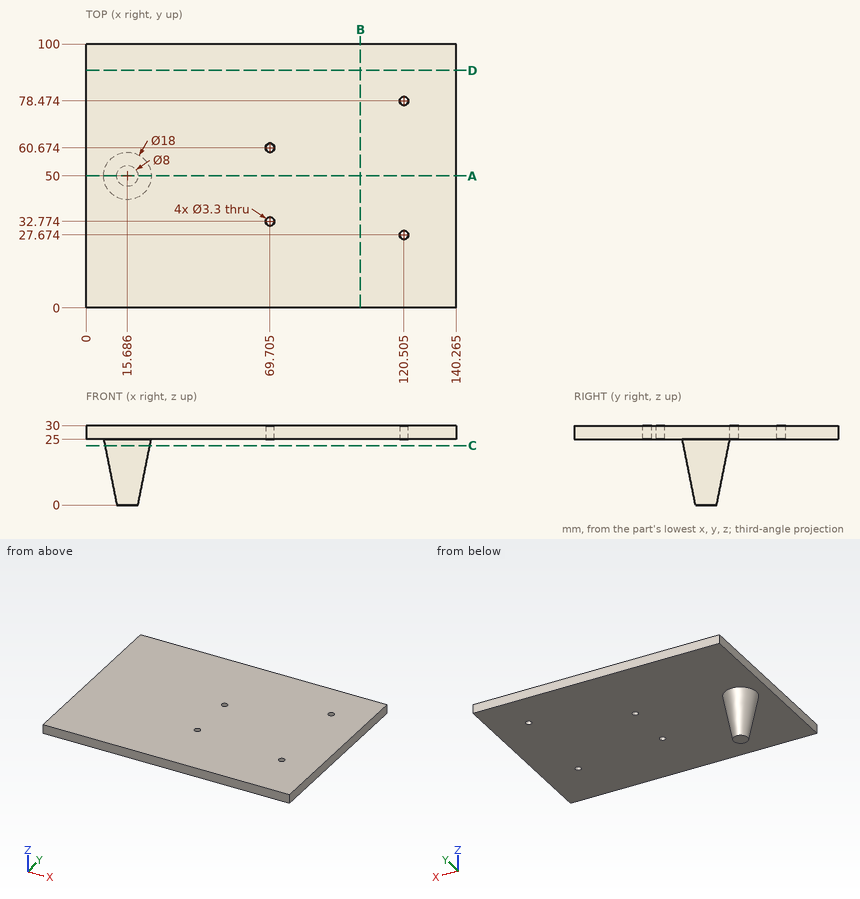
Geometry: see drawing. Coordinates: mm, zero at the bounding-box minimum. Give positions to 0.01 mm unless a question says otherwise; leave off trailing zeros. Order: outer loops, then holes, each group sorted by start corner. A loop starts at its lowest first (then second) coordinate and runs counter-clockwise, first axis right, second up.
1. Line query: probe 1 along Z at (x, y) = (56, 67); probe 2 along X at (y, z) = (34, 28) (1 decimal). Output: solid intervals per line, ascending.
Computed:
probe 1: z = 25 to 30
probe 2: x = 0 to 68.6, 70.8 to 140.3
2. Cut plane A-A (y = 50). Return loops of the section in (x, z) (1 decimal), and give its area (3 significant figures).
Computed:
outline: (0, 25) - (6.7, 25) - (11.7, 0) - (19.7, 0) - (24.7, 25) - (140.3, 25) - (140.3, 30) - (0, 30) - close
area: 1,030 mm2
3. Cut plane D-D (y = 90). Return loops of the section in (x, z) (1 decimal).
Computed:
outline: (0, 25) - (140.3, 25) - (140.3, 30) - (0, 30) - close
4. Cut plane B-B (x = 104). Return loops of the section in (y, z), and give its area (3 significant figures).
Computed:
outline: (0, 25) - (100, 25) - (100, 30) - (0, 30) - close
area: 500 mm2
5. Pin query (flat end, axial travel): pin 1 Ø10 at (y, z) = (59, 9) entering from +X; pin 2 Ø4.5 at (x, y) = (69.71, 60.67) entering from -Z. Return the tip coordinate at first contact, or that it passes through.
Computed:
pin 1: stops at x = 20.08
pin 2: stops at z = 25
6. Cut plane C-C (z = 22.5). Return loops of the section in (x, y) (1 decimal), and give its area (3 significant figures).
Computed:
outline: circle Ø17 at (15.7, 50)
area: 227 mm2
